Autodesk Inventor part; units mm, degrees
ref_plane "作業平面1" through (0, 0, 54) normal (0, 0, 1) x (1, 0, 0)
ref_plane "YZ Plane" through (0, 0, 0) normal (1, 0, 0) x (0, 1, 0)
ref_plane "XZ Plane" through (0, 0, 0) normal (0, 1, 0) x (-1, 0, 0)
sketch "スケッチ1" plane through (0, 0, 0) normal (0, 0, 1) x (1, 0, 0)
  circle A0 centre (0, 0) radius 3
  circle A1 centre (0, 0) radius 1.5
  dimension "d0" = 6
  dimension "d1" = 3
extrude "押し出し1" add sketch "スケッチ1" along normal blind 60
sketch "スケッチ2" plane through (0, 0, 60) normal (0, 0, 1) x (1, 0, 0)
  point P0 (0, 0)
ref_plane "作業平面1" through (0, 0, 54) normal (0, 0, 1) x (1, 0, 0)
sketch "スケッチ3" plane through (0, 0, 54) normal (0, 0, 1) x (1, 0, 0)
  circle A0 centre (0, 0) radius 3
  circle A1 centre (0, 0) radius 1.5
  dimension "d5" = 3
extrude "押し出し2" add sketch "スケッチ3" against normal blind 48 contours A1
properties part number "スペーサーm3-60　簡易筒型　売ってない" material "アルミニウム 2014-T4"
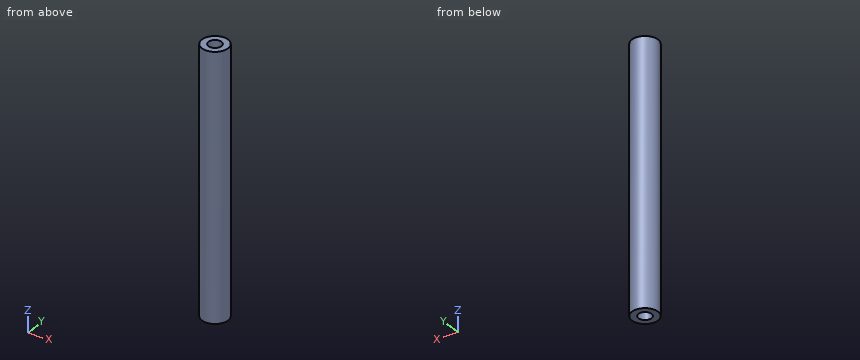
Source: CAD feature listing. Evaluate the final solid. Frame: model axes, mm. Give positions to 0.01 mm unless a question says otherwise; leave off trailing zeros. Loops run counter-clockwise (first coordinate to the right, second up) from the corner with the lowest first, then second, coordinate; pieces in that order, holes last. Notation, with made-up numbers: (63, -33) - (112, -33) arc R26 cw to (112, 0) - close; hole circle Ø11 at (44.25, 87.25). An arc over 180 degrees is marked (long way). Use CSV: the item, a comma, the result in double quotes.
1) Cut plane A-A (x = 0). Output: boundary loops of the cut face in (y, z), and give its area (3 significant figures).
Worked out:
outline,"(-3, 0) - (-1.5, 0) - (-1.5, 6) - (1.5, 6) - (1.5, 0) - (3, 0) - (3, 60) - (1.5, 60) - (1.5, 54) - (-1.5, 54) - (-1.5, 60) - (-3, 60) - close"
area,"324 mm^2"
2) Pin query (flat end, axial travel): P1, Ø1, axis at x = 1, z = 42, coming from the +Y side; P2, Ø1, axis at x = 0, y = -0.5, coming from the -Z side; P3, Ø3, axis at y = -2.5, z = 45.5, coming from the -X side; P4, Ø3.5, axis at x = 0, y = 0, coming from the +Z side. Return the tip coordinate at first contact, or that it passes through.
Worked out:
P1,"stops at y = 2.96"
P2,"stops at z = 6"
P3,"stops at x = -2.83"
P4,"stops at z = 60"
3) Line query: line 1 (Y direction, x = 0, z = 4); line 2 (Y direction, x = 2.6, z = 36); line 3 (X direction, y = 1.05, z = 55.5). Output: solid intervals per line, ascending.
Worked out:
line 1,"y = -3 to -1.5, 1.5 to 3"
line 2,"y = -1.5 to 1.5"
line 3,"x = -2.81 to -1.07, 1.07 to 2.81"
4) Cut plane D-D (y = -2.25). Output: boundary loops of the cut face in (x, z), and give its area (3 significant figures).
Worked out:
outline,"(-1.98, 0) - (1.98, 0) - (1.98, 60) - (-1.98, 60) - close"
area,"238 mm^2"
5) Cut plane C-C (z = 21). Output: boundary loops of the cut face in (x, y).
Worked out:
outline,"circle Ø6 at (0, 0)"
